Source: CAD feature listing. Evaluate the final solid. Frame: model axes, mm. A direction names the side the tool comes from. Give positions to 0.01 mm unless a question says otherwise; leave off trailing zeros. Order: outer loops, then holes, each group sorted by start corner. A loop starts at its lowest first (then second) coordinate and runs counter-clockwise, first axis right, second up. Notation, with made-up numbers: (8, 29) - (55, 29) arc R17 ccw to (55, 56) - close; hole circle Ø3 at (28.25, -9.5). An arc over 180 degrees is marked (long way). One line per item, written item: value. Start each with the question number.
from build123d import *

# Parameters (mm, degrees)
FILLET1_R          = 0.5
SKETCH2_R          = 1
CUT_EXTRUDE1_DEPTH = 16.588457268
FILLET2_R          = 0.1


with BuildPart() as part:
    # Sketch1 → Revolve1 (revolve)
    with BuildSketch(Plane(origin=(0, 0, 0), x_dir=(0, 0, -1), z_dir=(1, 0, 0)), mode=Mode.PRIVATE) as revolve1_sk:
        Polygon((0, 11), (0, 6), (0.8, 4.5), (0.8, 0), (1.8, 0), (1.8, 4.5), (1, 6), (1, 11), align=None)
    revolve(revolve1_sk.sketch.rotate(Axis((0, 0, 0), (0, 0, -1)), 90), axis=Axis((0, 0, 0), (0, 0, -1)))

    # Fillet1
    fillet1_edges = [part.edges().sort_by_distance(p)[0] for p in [
        (-6, 0, 0),
        (-4.5, 0, -1.8),
        (-6, 0, -1),
    ]]
    fillet(fillet1_edges, radius=FILLET1_R)

    # Sketch2 → Cut-Extrude1 (cut, through all)
    with BuildSketch(Plane(origin=(0, 0, -1), x_dir=(-1, 0, 0), z_dir=(0, 0, -1))):
        with Locations((6.363961031, 6.363961031)):
            Circle(SKETCH2_R)
        with Locations((6.363961031, -6.363961031)):
            Circle(SKETCH2_R)
        with Locations((-6.363961031, -6.363961031)):
            Circle(SKETCH2_R)
        with Locations((-6.363961031, 6.363961031)):
            Circle(SKETCH2_R)
    extrude(amount=-CUT_EXTRUDE1_DEPTH, mode=Mode.SUBTRACT)

    # Fillet2
    fillet2_edges = [part.edges().sort_by_distance(p)[0] for p in [
        (-11, 0, -1),
        (-11, 0, 0),
    ]]
    fillet(fillet2_edges, radius=FILLET2_R)


solid = part.part
1. Set-up query: faces 4 (the flat face through (0, 0, -1.8)), 5 (the flat face through (0, 0, -0.8)), 6 (the flat face through (-5, 5, -1)). Return all of +Z, -Z, +X, -X, +Y, -Y with unobstructed straight access to the full face (end or side cutting, diameter ignored); none if empty.
2. Section C-C on z = -0.5. Return the cut outline in (x, y) (1 decimal).
3. Contact query for flat-ended pins moving along their axis: pin 1 Ø2.5 at (x, y) = (-1, 1) entering from +Z; pin 2 Ø1.8 at (x, y) = (6.36, 6.36) entering from +Z; pin 3 Ø2 at (x, y) = (2, 6.5) entering from -Z. Output: stop coordinate, or through.
4. Section A-A on x = 0. Return the cut outline in (y, z) (3 decimals), then the cut area to 3 significant figures.
5. Section D-D on x = 6.75. Count the separate pieces of the cut face and the enclosed holes in it, then the cut area to 3 significant figures.
6. Draft query along X for faces 1 (the flat face through (5, 5, 0)), 2 (the cylindrical face through (5.41, 6.66, -0.51)), 3 (the cylindrical face through (-2.38, 10.74, -0.49)). Return one class per face: pulls with the +X half, pulls with the -X half, needs draft (parallel to the pull), parting line crosses it, or undercut.
7. Ray query, L1, parallel to X at y = -7, z = -0.95; L2, parallel to Z at x = 1.75, y = 2.5; L3, parallel to Z at x = -4.25, y = 6. Return the intervals inside material, ascending.
Data:
1. face 4: -Z, +X, -X, +Y, -Y
1. face 5: +Z
1. face 6: -Z
2. outline: circle Ø22 at (0, 0); hole circle Ø2 at (-6.4, -6.4); hole circle Ø2 at (-6.4, 6.4); hole circle Ø10.1 at (0, 0); hole circle Ø2 at (6.4, -6.4); hole circle Ø2 at (6.4, 6.4)
3. pin 1: stops at z = -0.8
3. pin 2: passes through
3. pin 3: stops at z = -1.11
4. outline: (-11, -0.9) arc R0.1 ccw to (-10.9, -1) - (-6.125, -1) arc R0.5 cw to (-5.89, -1.059) - (-4.61, -1.741) arc R0.5 ccw to (-4.375, -1.8) - (4.375, -1.8) arc R0.5 ccw to (4.61, -1.741) - (5.89, -1.059) arc R0.5 cw to (6.125, -1) - (10.9, -1) arc R0.1 ccw to (11, -0.9) - (11, -0.1) arc R0.1 ccw to (10.9, 0) - (6.125, 0) arc R0.5 ccw to (5.89, -0.059) - (4.5, -0.8) - (-4.5, -0.8) - (-5.89, -0.059) arc R0.5 ccw to (-6.125, 0) - (-10.9, 0) arc R0.1 ccw to (-11, -0.1) - close
4. area: 22.0 mm2
5. separate pieces: 3
5. enclosed holes: 0
5. area: 13.7 mm2
6. face 1: needs draft
6. face 2: undercut
6. face 3: parting line crosses it
7. L1: x = -8.47 to -7.14, -5.59 to 5.59, 7.14 to 8.47
7. L2: z = -1.8 to -0.8
7. L3: z = -1 to 0
